from build123d import *
from OCP.BRepFilletAPI import BRepFilletAPI_MakeChamfer

# Parameters (mm, degrees)
EXTRUDE_2_DEPTH     = 50
CHAMFER_1_SIZE      = 30
CHAMFER_2_SIZE      = 5
CHAMFER_3_SIZE      = 5
EXTRUDE_3_DEPTH     = 67
CHAMFER_6_SIZE      = 8
CHAMFER_6_SIZE2     = 6.474308837
CHAMFER_7_SIZE      = 59.001285691
CHAMFER_7_SIZE_2    = 8
CHAMFER_8_SIZE      = 59.001285691
CHAMFER_8_SIZE_2    = 8
EXTRUDE_4_DEPTH     = 5
CHAMFER_9_SIZE      = 13.737387097
CHAMFER_9_SIZE_2    = 5
SKETCH_5_R          = 1.1
CUT_EXTRUDE_1_DEPTH = 20


with BuildPart() as part:
    # Эскиз2 → Бобышка-Вытянуть2 (new body)
    with BuildSketch(Plane.XY):
        Polygon((-228.822789272, 61.401300251), (-228.822789272, 153.401300251), (-196.822789272, 185.401300251), (-129.822789272, 185.401300251), (-97.822789272, 153.401300251), (-97.822789272, 61.530932705), (-89.822789272, 61.530932705), (-89.822789272, 153.401300251), (-129.822789272, 193.401300251), (-196.822789272, 193.401300251), (-236.822789272, 153.401300251), (-236.822789272, 61.401300251), align=None)
    extrude(amount=EXTRUDE_2_DEPTH)

    # Фаска1
    chamfer_1_edges = [part.edges().sort_by_distance(p)[0] for p in [
        (-93.822789272, 61.530932705, 50),
        (-232.822789272, 61.401300251, 50),
    ]]
    chamfer(chamfer_1_edges, length=CHAMFER_1_SIZE)

    # Фаска2
    chamfer_2_edges = [part.edges().sort_by_distance(p)[0] for p in [
        (-109.822789272, 173.401300251, 50),
        (-89.822789272, 122.466116478, 50),
        (-163.322789272, 193.401300251, 50),
        (-216.822789272, 173.401300251, 50),
        (-236.822789272, 122.401300251, 50),
    ]]
    chamfer(chamfer_2_edges, length=CHAMFER_2_SIZE)

    # Фаска3
    chamfer_3_edges = [part.edges().sort_by_distance(p)[0] for p in [
        (-97.822789272, 76.530932705, 35),
        (-228.822789272, 76.401300251, 35),
    ]]
    chamfer(chamfer_3_edges, length=CHAMFER_3_SIZE)

    # Эскиз3 → Бобышка-Вытянуть3 (add)
    with BuildSketch(Plane(origin=(-129.822789272, 0, 0), x_dir=(0, 0, -1), z_dir=(1, 0, 0))):
        Polygon((-45, 193.401300251), (0, 193.401300251), (0, 200.504313431), align=None)
    extrude(amount=-EXTRUDE_3_DEPTH)

    # Фаска6: one chamfer whose edges measure the first distance from different faces: ONE call of the kernel's chamfer builder (chamfer() names one face for all edges)
    chamfer_6_edges_1 = [part.edges().sort_by_distance(p)[0] for p in [
        (-97.822789272, 153.401300251, 25),
    ]]
    chamfer_6_side_1 = [part.faces().sort_by_distance(p)[0] for p in [
        (-113.822789272, 169.401300251, 25),
    ]]
    chamfer_6_edges_2 = [part.edges().sort_by_distance(p)[0] for p in [
        (-228.822789272, 153.401300251, 25),
    ]]
    chamfer_6_side_2 = [part.faces().sort_by_distance(p)[0] for p in [
        (-228.822789272, 113.309285826, 22.779788417),
    ]]
    chamfer_6 = BRepFilletAPI_MakeChamfer(part.part.solid().wrapped)
    for e in chamfer_6_edges_1:
        chamfer_6.Add(CHAMFER_6_SIZE, CHAMFER_6_SIZE2, e.wrapped, chamfer_6_side_1[0].wrapped)  # the first distance lies on this face
    for e in chamfer_6_edges_2:
        chamfer_6.Add(CHAMFER_6_SIZE, CHAMFER_6_SIZE2, e.wrapped, chamfer_6_side_2[0].wrapped)  # the first distance lies on this face
    add(Compound.cast(chamfer_6.Shape()), mode=Mode.REPLACE)

    # Фаска7
    # the kernel refuses this chamfer: 59.001285691, 8 mm, written as the material it adds along each edge
    with BuildSketch(Plane(origin=(-196.822789272, 193.401300251, 0), x_dir=(-0.7047321498610482, -0.7094734645863968, 0), z_dir=(0, 0, 1))) as chamfer_7_piece_1_section:
        Polygon((CHAMFER_7_SIZE * 0.999994379973, -CHAMFER_7_SIZE * 0.00335261579405), (-CHAMFER_7_SIZE_2 * 0.709473464586, -CHAMFER_7_SIZE_2 * 0.704732149861), (0, 0), align=None)
    chamfer_7_piece_1 = extrude(amount=198.381753037, mode=Mode.PRIVATE)
    chamfer_7_piece_1 = split(chamfer_7_piece_1, bisect_by=Plane(origin=(-220.880283212, 186.62893037, 32.777571564), z_dir=(0.49999999999999994, -0.5, -0.7071067811865477)), keep=Keep.TOP, mode=Mode.PRIVATE)
    chamfer_7_piece_1 = split(chamfer_7_piece_1, bisect_by=Plane(origin=(-236.822789272, 178.689900101, 21.550087285), z_dir=(1, 0, 0)), keep=Keep.TOP, mode=Mode.PRIVATE)
    chamfer_7_piece_1 = split(chamfer_7_piece_1, bisect_by=Plane(origin=(-212.941252942, 196.655142254, 24.385806214), z_dir=(1.0444770759811184e-15, -0.9877705725829901, -0.1559143865686293)), keep=Keep.TOP, mode=Mode.PRIVATE)
    add(chamfer_7_piece_1)

    # Фаска8
    # the kernel refuses this chamfer: 59.001285691, 8 mm, written as the material it adds along each edge
    with BuildSketch(Plane(origin=(-129.822789272, 193.401300251, 0), x_dir=(0.7047321498610463, -0.7094734645863986, 0), z_dir=(0, 0, 1))) as chamfer_8_piece_1_section:
        Polygon((CHAMFER_8_SIZE * 0.999994379973, CHAMFER_8_SIZE * 0.00335261579405), (-CHAMFER_8_SIZE_2 * 0.709473464586, CHAMFER_8_SIZE_2 * 0.704732149861), (0, 0), align=None)
    chamfer_8_piece_1 = extrude(amount=198.381753037, mode=Mode.PRIVATE)
    chamfer_8_piece_1 = split(chamfer_8_piece_1, bisect_by=Plane(origin=(-89.822789272, 178.689900101, 21.550087285), z_dir=(-1, 0, 0)), keep=Keep.TOP, mode=Mode.PRIVATE)
    chamfer_8_piece_1 = split(chamfer_8_piece_1, bisect_by=Plane(origin=(-105.765295333, 186.62893037, 32.777571565), z_dir=(-0.5000000000000016, -0.4999999999999975, -0.7071067811865482)), keep=Keep.TOP, mode=Mode.PRIVATE)
    chamfer_8_piece_1 = split(chamfer_8_piece_1, bisect_by=Plane(origin=(-113.704325602, 196.655142254, 24.385806214), z_dir=(0, -0.9877705725829332, -0.15591438656898948)), keep=Keep.TOP, mode=Mode.PRIVATE)
    add(chamfer_8_piece_1)

    # Эскиз4 → Бобышка-Вытянуть4 (add)
    with BuildSketch(Plane(origin=(0, 0, 0), x_dir=(-1, 0, 0), z_dir=(0, 0, -1))):
        Polygon((97.822789272, 146.926991414), (102.822789272, 130.926991414), (102.822789272, 61.530932705), (97.822789272, 61.530932705), align=None)
        Polygon((228.822789272, 145.401300251), (228.822789272, 61.530932705), (223.822789272, 61.530932705), (223.822789272, 130.926991414), align=None)
    extrude(amount=-EXTRUDE_4_DEPTH)

    # Фаска9
    # the kernel refuses this chamfer: 13.737387097, 5 mm, written as the material it adds along each edge
    with BuildSketch(Plane(origin=(-97.822789272, 61.530932705, 5), x_dir=(0.013184058198649358, 0, 0.9999130865277315), z_dir=(0, 1, 0))) as chamfer_9_piece_1_section:
        Polygon((CHAMFER_9_SIZE * 0.999913086548, -CHAMFER_9_SIZE * 0.0131840581989), (-CHAMFER_9_SIZE_2 * 0.0131840581986, -CHAMFER_9_SIZE_2 * 0.999913086528), (0, 0), align=None)
    chamfer_9_piece_1 = extrude(amount=121.033515956, mode=Mode.PRIVATE)
    chamfer_9_piece_1 = split(chamfer_9_piece_1, bisect_by=Plane(origin=(-114.063470216, 91.772466116, 20.202674346), z_dir=(0.7071067811865477, 0.5, -0.4999999999999999)), keep=Keep.TOP, mode=Mode.PRIVATE)
    chamfer_9_piece_1 = split(chamfer_9_piece_1, bisect_by=Plane(origin=(-110.682470029, 105.776012992, 9.758348452), z_dir=(0.9544799780350295, -0.2982749931359476, 0)), keep=Keep.TOP, mode=Mode.PRIVATE)
    chamfer_9_piece_1 = split(chamfer_9_piece_1, bisect_by=Plane(origin=(-102.822789272, 102.21679201, 9.758348452), z_dir=(1, 0, 0)), keep=Keep.TOP, mode=Mode.PRIVATE)
    add(chamfer_9_piece_1)
    with BuildSketch(Plane(origin=(-228.822789272, 181.038757498, 5), x_dir=(0.9950833631817486, 0, -0.09904090225205033), z_dir=(0, -1, 0))) as chamfer_9_piece_2_section:
        Polygon((CHAMFER_9_SIZE_2 * 0.995083363182, CHAMFER_9_SIZE_2 * 0.0990409022521), (-CHAMFER_9_SIZE * 0.099040902254, CHAMFER_9_SIZE * 0.995083363202), (0, 0), align=None)
    chamfer_9_piece_2 = extrude(amount=119.507824793, mode=Mode.PRIVATE)
    chamfer_9_piece_2 = split(chamfer_9_piece_2, bisect_by=Plane(origin=(-199.458401516, 124.497296703, 34.497413224), z_dir=(-0.7071067811865471, 0.5000000000000006, -0.5000000000000001)), keep=Keep.TOP, mode=Mode.PRIVATE)
    chamfer_9_piece_2 = split(chamfer_9_piece_2, bisect_by=Plane(origin=(-228.851428884, 145.484207968, 13.577093316), z_dir=(-0.945194554128901, -0.32650766429759087, 0)), keep=Keep.TOP, mode=Mode.PRIVATE)
    chamfer_9_piece_2 = split(chamfer_9_piece_2, bisect_by=Plane(origin=(-223.822789272, 145.417616611, 13.577093316), z_dir=(-1, 0, 0)), keep=Keep.TOP, mode=Mode.PRIVATE)
    add(chamfer_9_piece_2)

    # Эскиз5 → Вырез-Вытянуть1 (cut)
    with BuildSketch(Plane(origin=(0, 0, 0), x_dir=(-1, 0, 0), z_dir=(0, 0, -1))):
        with Locations((96.322789272, 86.530932705)):
            Circle(SKETCH_5_R)
        with Locations((230.322789272, 86.530932705)):
            Circle(SKETCH_5_R)
        with Locations((163.322789272, 192.952806841)):
            Circle(SKETCH_5_R)
    extrude(amount=-CUT_EXTRUDE_1_DEPTH, mode=Mode.SUBTRACT)


solid = part.part
Read the model definition and answer for the solid it produces. Units are mm, in the model's axes. A direction names the side the tool comes from. Coordinates: 2 decimals unless noted, no trailing zeros. Loops run counter-clockwise (first coordinate to the right, second up) from the corner with the lowest first, then second, coordinate; pieces in that order, holes last.
Q1. The mould has two halves that part along X. Classify faces 1 (the face through (-214.33, 175.06, 45.59)), 2 (the face through (-210.726, 171.498, 24.65)), 3 (the face through (-164, 188, 0)): +X half, -X half, draft (parallel to the pull), parting line (faces both ways), or undercut.
Q2. Each of these flat-tipped pins is pushed along its axis until it touches: pin 1 Ø2 at (x, z) = (-105, 17) entering from +Y; pin 2 Ø6 at (y, z) = (162.5, 6) entering from -X; pin 3 Ø14.5 at (x, z) = (-98, 9.5) entering from -Y. Where does it stop, or does it pass through?
Q3. The part is cut by section C-C on x = -169. Write down the section's boundary in (y, z).
Q4. The part is cut by section D-D on z = 9.5. Write down the section's boundary in (x, y).
Q5. The part is cut by section B-B on z = 26. Write down the section's boundary in (x, y).
Q6. Which of the six approach directions +Z, -Z, +X, -X, +Y, -Y give full straight-line access (tool end or side, diameter ignored) to faces 4 (the face through (-95, 61.531, 8)), 5 (the face through (-226.5, 151.78, 24.65)), 6 (the face through (-116.836, 172.414, 24.65))?
Q7. The part is cut by section A-A on y = 118. Write down the section's boundary in (x, z).
Q8. Consider probe 1 along X at (y, z) = (88, 19.5); probe 2 along X at (y, z) = (89, 7.5); probe 3 along X at (y, z) = (87, 13). Determine where each line is inside the solid, lowest interval first.
Results below:
1. face 1: -X half
1. face 2: undercut
1. face 3: draft
2. pin 1: stops at y = 173.01
2. pin 2: stops at x = -231.98
2. pin 3: stops at y = 61.53
3. outline: (185.4, 0) - (200.5, 0) - (193.4, 45) - (188.4, 50) - (185.4, 50) - close
4. outline: (-236.82, 61.4) - (-228.82, 61.4) - (-228.82, 61.53) - (-226.31, 61.53) - (-225.46, 62.73) - (-225.46, 135.67) - (-228.82, 145.4) - (-224.24, 157.98) - (-196.82, 185.4) - (-129.82, 185.4) - (-103.48, 159.06) - (-97.82, 146.93) - (-101.18, 136.17) - (-101.18, 62.86) - (-100.25, 61.53) - (-89.82, 61.53) - (-89.82, 153.73) - (-127.81, 199) - (-198.83, 199) - (-236.82, 153.73) - close; hole circle Ø2.2 at (-230.32, 86.53); hole circle Ø2.2 at (-163.32, 192.95); hole circle Ø2.2 at (-96.32, 86.53)
5. outline: (-236.82, 67.4) - (-233.82, 67.4) - (-228.82, 74.47) - (-228.82, 145.4) - (-224.24, 157.98) - (-196.82, 185.4) - (-129.82, 185.4) - (-103.48, 159.06) - (-97.82, 146.93) - (-97.82, 74.6) - (-92.82, 67.53) - (-89.82, 67.53) - (-89.82, 153.73) - (-125.63, 196.4) - (-201.02, 196.4) - (-236.82, 153.73) - close
6. face 4: +Z, -Z, +X, -Y
6. face 5: +Z, -Z
6. face 6: +Z, -Z, -Y
7. outline: (-236.82, 0) - (-223.82, 0) - (-223.82, 5) - (-228.82, 18.74) - (-228.82, 50) - (-231.82, 50) - (-236.82, 45) - close; (-102.82, 0) - (-89.82, 0) - (-89.82, 45) - (-94.82, 50) - (-97.82, 50) - (-97.82, 18.74) - (-102.82, 5) - close
8. probe 1: x = -236.82 to -228.82, -97.82 to -89.82
8. probe 2: x = -236.82 to -224.73, -101.91 to -89.82
8. probe 3: x = -236.82 to -231.32, -229.33 to -226.73, -99.91 to -97.32, -95.33 to -89.82
